Source: CAD feature listing. Evaluate the final solid. Frame: model axes, mm. A direction names the side the tool comes from. Round coordinates to 2 decimals unless told otherwise and drop trailing zeros. Order: outer loops, then holes, each group sorted by start corner. A loop starts at its lowest first (then second) coordinate and runs counter-clockwise, first axis right, second up. Notation, with made-up numbers: (60, 39) - (90, 39) arc R24 cw to (90, 53) - close; hole circle Ø6 at (86, 56). An arc over 180 degrees is marked (long way). Put each result on its own line as item: value. Start each with the question number.
1) Section B-B on z = -54.5. Output: boundary loops of the cut face in (x, y).
2) Contact query for flat-ended pins moving along their axis: P1, Ø6.5, axis at x = -15.5, z = -69.5, coming from the -Y side; P2, Ø3, axis at x = -23.5, z = -60.5, coming from the +Y side; P3, Ø3.5, axis at y = 5.5, z = -34, coming from the +X side; P4, Ø15, axis at x = -138.2, z = -68.2, coming from the +Y side. Output: stop coordinate, or through.
3) Section D-D on z = -15. Output: boundary loops of the cut face in (x, y), then the cut area to 3 significant figures.
4) Section C-C on x = -138.2. Output: boundary loops of the cut face in (y, z).
5) Access query for faces 1 (the face through (-144.694, 0.296, -67.914)), 2 (the face through (-22, 7, -59)), 3 (the face through (-76, 8.6, -1)). Directions: +Z, -Z, +X, -X, +Y, -Y. A direction counts if a zero-diameter tool reaches every point of the face in a straight line with its end or side. Return the directions, or none.
6) Section A-A on y = 4.5. State how many separate pieces and enclosed holes the cut face has, then the cut area to 3 significant figures.
7) Line query: probe 1 along X at (y, z) = (2.6, -22.6); probe 2 along Z at (x, y) = (-80.05, 5.8); probe 3 along X at (y, z) = (3.5, -64.5). Output: solid intervals per line, ascending. Write a range as [from, to].
8) Mould query, pull axis X, two halves, no side actions, for faces 4 (the face through (-76, 5, 0)), 5 (the face through (0, 5, -42)), 6 (the face through (-15, 0.6, -15)). Classes: +X half, -X half, draft (parallel to the pull), parting line (faces both ways), or undercut.
Autodesk Inventor part; units mm, degrees
ref_plane "YZ Plane" through (0, 0, 0) normal (1, 0, 0) x (0, 1, 0)
ref_plane "XZ Plane" through (0, 0, 0) normal (0, 1, 0) x (-1, 0, 0)
ref_plane "XY Plane" through (0, 0, 0) normal (0, 0, 1) x (1, 0, 0)
sketch "Skizze1" plane through (0, 0, 0) normal (0, 1, 0) x (-1, 0, 0)
  line L0 (0, 0) -> (153.2, 0)
  line L1 (153.2, 0) -> (153.2, -83.2)
  line L2 (153.2, -83.2) -> (0, -83.2)
  line L3 (0, -83.2) -> (0, 0)
  dimension "d0" = 153.2
  dimension "d1" = 83.2
extrude "Extrusion1" add sketch "Skizze1" along normal blind 8.6
sketch "Skizze2" plane through (0, 8.6, 0) normal (0, 1, 0) x (1, 0, 0)
  line L0 (-1.5, 1.5) -> (-151.7, 1.5)
  line L1 (-151.7, 1.5) -> (-151.7, 81.7)
  line L2 (-151.7, 81.7) -> (-1.5, 81.7)
  line L3 (-1.5, 81.7) -> (-1.5, 1.5)
  line L4 (-153.2, 0) -> (0, 0)
  line L5 (0, 83.2) -> (-153.2, 83.2)
  line L6 (0, 0) -> (0, 83.2)
  line L7 (-153.2, 83.2) -> (-153.2, 0)
  dimension "d4" = 1.5
  dimension "d5" = 1.5
  dimension "d6" = 1.5
  dimension "d7" = 1.5
extrude "Extrusion2" cut sketch "Skizze2" against normal blind 7.1 contours L0 L1 L2 L3
sketch "Skizze4" plane through (0, 1.5, 0) normal (0, 1, 0) x (1, 0, 0)
  circle A0 centre (-80.05, 22.6) radius 2.75
  circle A1 centre (-80.05, 60.6) radius 2.75
  circle A2 centre (-23.05, 22.6) radius 2.75
  circle A3 centre (-23.05, 60.6) radius 2.75
  circle A4 centre (-80.05, 22.6) radius 1.2
  circle A5 centre (-80.05, 60.6) radius 1.2
  circle A6 centre (-23.05, 22.6) radius 1.2
  circle A7 centre (-23.05, 60.6) radius 1.2
  line L0 (-1.5, 81.7) -> (-1.5, 1.5)
  line L1 (-1.5, 1.5) -> (-151.7, 1.5)
  line L2 (-151.7, 81.7) -> (-1.5, 81.7)
  point P0 (0, 0)
  dimension "d13" = 5.5
  dimension "d14" = 5.5
  dimension "d15" = 5.5
  dimension "d16" = 5.5
  dimension "d17" = 38
  dimension "d18" = 38
  dimension "d19" = 57
  dimension "d40" = 2.4
  dimension "d41" = 2.4
  dimension "d42" = 2.4
  dimension "d43" = 2.4
  dimension "d44" = 21.55
  dimension "d45" = 21.1
  dimension "d47" = 21.1
  dimension "d51" = 21.55
  dimension "d53" = 57
  dimension "d54" = 21.1
  dimension "d55" = 21.1
extrude "Extrusion4" add sketch "Skizze4" along normal blind 5.5
fillet "Rundung1" radius 2 4 edges at (0, 4.3, 0) (0, 4.3, -83.2) (-153.2, 4.3, 0) (-153.2, 4.3, -83.2)
fillet "Rundung2" radius 2 8 edges at (-0.5858, 0, -0.5858) (0, 0, -41.6) (-0.5858, 0, -82.6142) (-76.6, 0, -83.2) (-152.6142, 0, -82.6142) (-153.2, 0, -41.6) (-152.6142, 0, -0.5858) (-76.6, 0, 0)
sketch "Skizze6" plane through (0, 0, 0) normal (0, -1, 0) x (1, 0, 0)
  circle A0 centre (-138.2, -68.2) radius 6.5
  circle A1 centre (-138.2, -15) radius 6.5
  circle A2 centre (-15, -68.2) radius 6.5
  circle A3 centre (-15, -15) radius 6.5
  line L0 (-2, 0) -> (-151.2, 0)
  line L1 (-151.2, -83.2) -> (-2, -83.2)
  line L2 (-153.2, -2) -> (-153.2, -81.2)
  line L3 (0, -81.2) -> (0, -2)
  point P0 (0, 0)
  dimension "d26" = 13
  dimension "d27" = 13
  dimension "d28" = 13
  dimension "d29" = 13
  dimension "d63" = 15
  dimension "d64" = 15
  dimension "d65" = 15
  dimension "d66" = 15
  dimension "d67" = 15
  dimension "d68" = 15
  dimension "d69" = 15
  dimension "d70" = 15
extrude "Extrusion6" cut sketch "Skizze6" against normal blind 0.6
properties part number "Datapad_Case_v2"
Answer sheet:
1. outline: (-153.2, 2) arc R2 ccw to (-151.2, 0) - (-2, 0) arc R2 ccw to (0, 2) - (0, 8.6) - (-1.5, 8.6) - (-1.5, 1.5) - (-151.7, 1.5) - (-151.7, 8.6) - (-153.2, 8.6) - close
2. P1: y = 0.6
2. P2: y = 7
2. P3: x = 0
2. P4: y = 1.5
3. outline: (-153.2, 2) arc R2 ccw to (-151.2, 0) - (-144.7, 0) - (-144.7, 0.6) - (-131.7, 0.6) - (-131.7, 0) - (-21.5, 0) - (-21.5, 0.6) - (-8.5, 0.6) - (-8.5, 0) - (-2, 0) arc R2 ccw to (0, 2) - (0, 8.6) - (-1.5, 8.6) - (-1.5, 1.5) - (-151.7, 1.5) - (-151.7, 8.6) - (-153.2, 8.6) - close
3. area: 234 mm^2
4. outline: (0, -81.2) arc R2 ccw to (2, -83.2) - (8.6, -83.2) - (8.6, -81.7) - (1.5, -81.7) - (1.5, -1.5) - (8.6, -1.5) - (8.6, 0) - (2, 0) arc R2 ccw to (0, -2) - (0, -8.5) - (0.6, -8.5) - (0.6, -21.5) - (0, -21.5) - (0, -61.7) - (0.6, -61.7) - (0.6, -74.7) - (0, -74.7) - close
5. face 1: -Y
5. face 2: +Y
5. face 3: +Z, -Z, +X, -X, +Y
6. separate pieces: 5
6. enclosed holes: 5
6. area: 774 mm^2
7. probe 1: [-153.2, -151.7], [-82.8, -81.25], [-78.85, -77.3], [-25.8, -24.25], [-21.85, -20.3], [-1.5, 0]
7. probe 2: [-83.2, -81.7], [-63.35, -61.8], [-59.4, -57.85], [-25.35, -23.8], [-21.4, -19.85], [-1.5, 0]
7. probe 3: [-153.2, -151.7], [-1.5, 0]
8. face 4: draft
8. face 5: +X half
8. face 6: undercut
